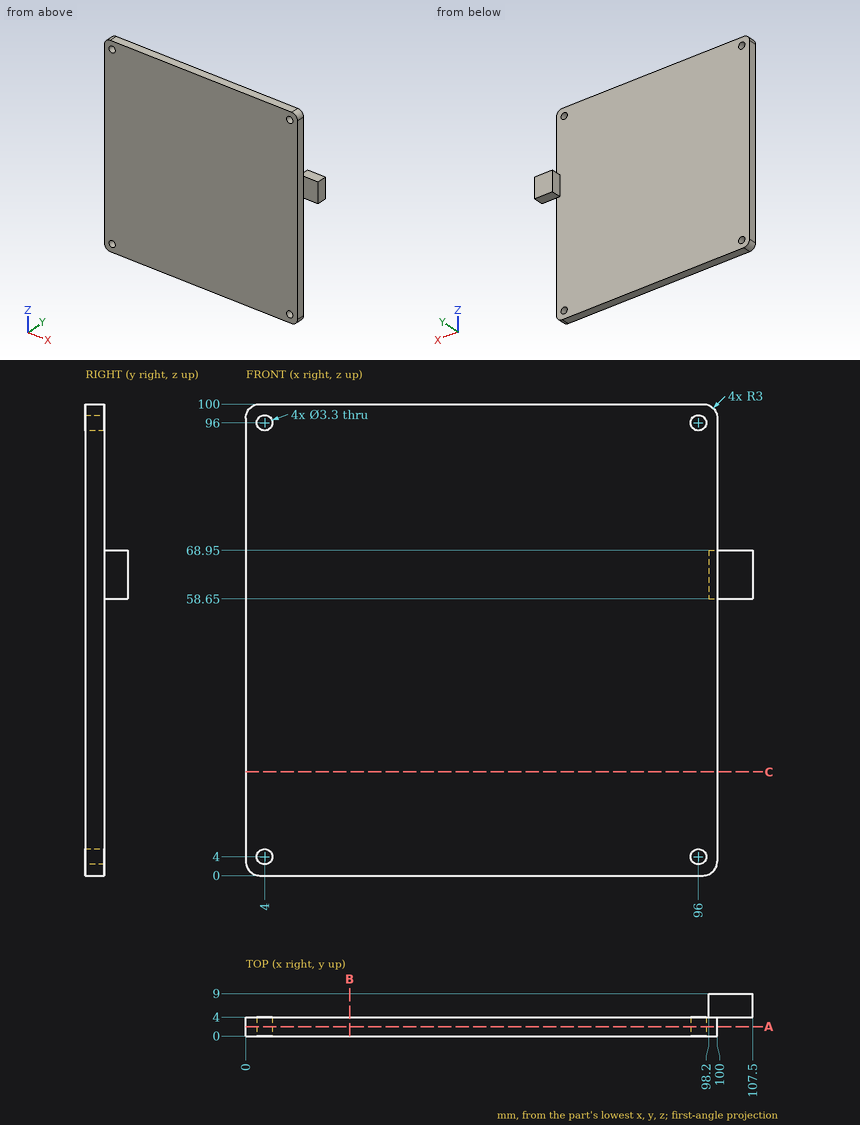
Job drawing, mm, ordinate dimensions from the low corner. One solid piece. Round coordinates to 2 decimals unless told otherwise and drop trailing zeros. Write each loop counter-clockwise with the first axis right and the second up, starting at its lowest first coordinate (ties: lowest second). Pieces come first, ordered by that corner, then holes.
1) Band-saw the part on B-B, the plane x = 22. List the corners of the cut face in (y, z), and give its area (3 significant figures).
2) Drill centre lines: probe 1 along X at (y, z) = (1.9, 4); probe 2 along Y at (x, z) = (26, 73.5); probe 3 along X at (y, z) = (1.5, 49.5). Where is each one in solid material? Low to high.
3) Pin check, flat tips, straight feed: pin 1 (1 mm diameter, centred on x = 69.5, z = 75.5, fed in from +Y); pin 2 (4.5 mm diameter, centred on y = 1, z = 29.5, fed in from +X); pin 3 (1.5 mm diameter, centred on y = 7.5, z = 66.5, fed in from -X). Stop position of each tip, or through.
4) Band-saw the part on A-A, the plane y = 2. List the corners of the cut face in (x, z), and give its area (3 significant figures).
5) Band-saw the part on C-C, the plane z = 22. List the corners of the cut face in (x, y).
Ans:
1. outline: (0, 0) - (4, 0) - (4, 100) - (0, 100) - close
1. area: 400 mm2
2. probe 1: x = 0 to 2.35, 5.65 to 94.35, 97.65 to 100
2. probe 2: y = 0 to 4
2. probe 3: x = 0 to 100
3. pin 1: stops at y = 4
3. pin 2: stops at x = 100
3. pin 3: stops at x = 98.2
4. outline: (0, 3) arc R3 ccw to (3, 0) - (97, 0) arc R3 ccw to (100, 3) - (100, 97) arc R3 ccw to (97, 100) - (3, 100) arc R3 ccw to (0, 97) - close; hole circle Ø3.3 at (4, 4); hole circle Ø3.3 at (4, 96); hole circle Ø3.3 at (96, 4); hole circle Ø3.3 at (96, 96)
4. area: 9,960 mm2
5. outline: (0, 0) - (100, 0) - (100, 4) - (0, 4) - close
